Can you work these out from the drawing? Everything is in mm from the part's minimum corner. Give positions to 0.01 mm unless a question says otherwise; leave off trailing zeros. Order: outer loops, then holes, each group sorted by start corner. A loop starts at its lowest first (then second) coordinate and runs counter-clockwise, first axis right, second up. Notation, with made-up numbers: (7, 75) -> (48, 75) arc R29 ccw to (48, 111) -> close; hole circle Ø7 at (-2, 60.5). An arc over 180 degrees is marked (long way). Answer as CSV lines item,"result". Start each with the question number.
(1) I want a section at A-A (z = 241). Please give me the cut outline in (x, y), plus the area to 3 significant figures.
(2) I need wall thicknesses on L1, parallel to Z at x = 50, y = 6; L2, parallel to X at y = 1.5, z = 300; L3, parallel to X at y = 6.25, z = 250.5. Which ranges of each line are inside material? Lowest first, please.
(3) I want a section at B-B (x = 81.5). Please give me the cut outline in (y, z).
(4) I want a section at C-C (y = 4.5). Please give me the cut outline in (x, z), plus the area to 3 significant figures.
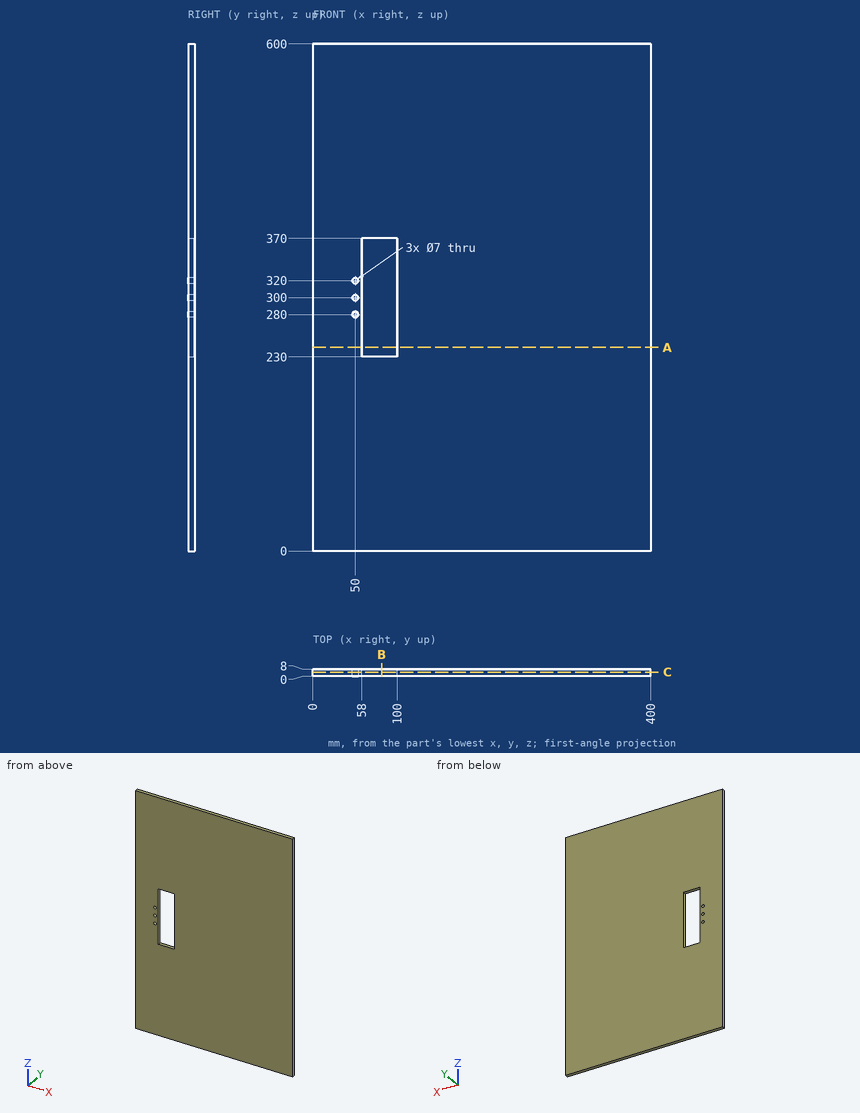
Final values:
1,outline,"(0, 0) -> (58, 0) -> (58, 8) -> (0, 8) -> close; (100, 0) -> (400, 0) -> (400, 8) -> (100, 8) -> close"
1,area,"2,860 mm²"
2,L1,"0 to 276.5, 283.5 to 296.5, 303.5 to 316.5, 323.5 to 600"
2,L2,"0 to 46.5, 53.5 to 58, 100 to 400"
2,L3,"0 to 58, 100 to 400"
3,outline,"(0, 0) -> (8, 0) -> (8, 230) -> (0, 230) -> close; (0, 370) -> (8, 370) -> (8, 600) -> (0, 600) -> close"
4,outline,"(0, 0) -> (400, 0) -> (400, 600) -> (0, 600) -> close; hole circle Ø7 at (50, 280); hole circle Ø7 at (50, 300); hole circle Ø7 at (50, 320); hole (58, 230) -> (100, 230) -> (100, 370) -> (58, 370) -> close"
4,area,"234,000 mm²"
